from build123d import *

# Parameters (mm, degrees)
SKETCH1_R                      = 27.4955
SKETCH1_R_2                    = 2
SKETCH1_R_3                    = 52.3875
SKETCH1_R_4                    = 3.3
BOSS_EXTRUDE1_DEPTH            = 9.525
M8_CLEARANCE_HOLE1_D           = 9
M8_CLEARANCE_HOLE1_CSINK_D     = 9.05
M8_CLEARANCE_HOLE1_CSINK_ANGLE = 90
CIRPATTERN1_COUNT              = 9
CUT_EXTRUDE2_DEPTH             = 705.952403184


with BuildPart() as part:
    # Sketch1 → Boss-Extrude1 (new body)
    with BuildSketch(Plane(origin=(0, 0, 0), x_dir=(-1, 0, 0), z_dir=(0, 1, 0))):
        with BuildLine():
            Line((-663.918846707, 4.476573271), (-466.57213203, 18.457038772))
            ThreePointArc((-466.57213203, 18.457038772), (-464.265511177, 17.802436421), (-462.085988967, 16.80309317))
            ThreePointArc((-462.085988967, 16.80309317), (-454.417575787, 16.107140218), (-448.740207572, 21.308717033))
            Line((-448.740207572, 21.308717033), (-396.041564291, 141.567674451))
            ThreePointArc((-396.041564291, 141.567674451), (-393.869824608, 172.384252636), (-411.692336104, 197.617881552))
            ThreePointArc((-411.692336104, 197.617881552), (-413.372500119, 198.071242365), (-414.950136715, 197.336701751))
            Line((-414.950136715, 197.336701751), (-420.215020333, 192.071818133))
            ThreePointArc((-420.215020333, 192.071818133), (-427.298656721, 190.662795249), (-431.31121441, 196.668012211))
            Line((-431.31121441, 196.668012211), (-431.31121441, 203.240745001))
            ThreePointArc((-431.31121441, 203.240745001), (-431.968379704, 204.945600851), (-433.59982344, 205.768273949))
            ThreePointArc((-433.59982344, 205.768273949), (-438.15, 205.994), (-442.70017656, 205.768273949))
            ThreePointArc((-442.70017656, 205.768273949), (-444.331620296, 204.945600851), (-444.98878559, 203.240745001))
            Line((-444.98878559, 203.240745001), (-444.98878559, 196.668012211))
            ThreePointArc((-444.98878559, 196.668012211), (-451.48878559, 190.168012211), (-457.98878559, 196.668012211))
            Line((-457.98878559, 196.668012211), (-457.98878559, 197.245022653))
            ThreePointArc((-457.98878559, 197.245022653), (-459.278285753, 199.455870942), (-461.837486501, 199.421924563))
            ThreePointArc((-461.837486501, 199.421924563), (-464.019895008, 198.024699819), (-466.120112298, 196.506730383))
            Line((-466.120112298, 196.506730383), (-526.629683433, 150.121113421))
            ThreePointArc((-526.629683433, 150.121113421), (-551.530592574, 139.247052869), (-578.312485484, 134.661130809))
            ThreePointArc((-578.312485484, 134.661130809), (-599.244289514, 129.920579306), (-617.300018038, 118.318686532))
            ThreePointArc((-617.300018038, 118.318686532), (-626.772573796, 112.207783301), (-637.753125569, 109.658286556))
            Line((-637.753125569, 109.658286556), (-662.485690794, 106.73386739))
            ThreePointArc((-662.485690794, 106.73386739), (-670.168377129, 100.916938085), (-668.842832121, 91.372134981))
            Line((-668.842832121, 91.372134981), (-653.346537148, 71.746276485))
            ThreePointArc((-653.346537148, 71.746276485), (-651.347572908, 64.158994024), (-653.346537148, 56.571711562))
            Line((-653.346537148, 56.571711562), (-673.057822329, 18.34288652))
            ThreePointArc((-673.057822329, 18.34288652), (-672.544957076, 8.73610108), (-663.918846707, 4.476573271))
        make_face()
        with Locations(Location((-438.15, 160.02, 0), (0, 0, 270))):
            Circle(SKETCH1_R, mode=Mode.SUBTRACT)
        with Locations(Location((-632.402453753, 70.257452317, 0), (0, 0, 270))):
            Circle(SKETCH1_R_2, mode=Mode.SUBTRACT)
        with Locations(Location((-575.31, 72.821477372, 0), (0, 0, 270))):
            Circle(SKETCH1_R_3, mode=Mode.SUBTRACT)
        with Locations(Location((-661.367230642, 97.274762153, 0), (0, 0, 270))):
            Circle(SKETCH1_R_4, mode=Mode.SUBTRACT)
        with Locations(Location((-664.591931322, 13.977761728, 0), (0, 0, 270))):
            Circle(SKETCH1_R_4, mode=Mode.SUBTRACT)
        with Locations(Location((-457.464330992, 25.131712658, 0), (0, 0, 270))):
            Circle(SKETCH1_R_4, mode=Mode.SUBTRACT)
        with BuildLine():
            ThreePointArc((-518.217546247, 72.257452317), (-520.217546247, 70.257452317), (-518.217546247, 68.257452317))
            ThreePointArc((-518.217546247, 68.257452317), (-516.217546247, 70.257452317), (-518.217546247, 72.257452317))
        make_face(mode=Mode.SUBTRACT)
        with BuildLine():
            ThreePointArc((-575.31, 17.671477372), (-577.31, 15.671477372), (-575.31, 13.671477372))
            ThreePointArc((-575.31, 13.671477372), (-573.31, 15.671477372), (-575.31, 17.671477372))
        make_face(mode=Mode.SUBTRACT)
        with BuildLine():
            ThreePointArc((-575.31, 131.971477372), (-577.31, 129.971477372), (-575.31, 127.971477372))
            ThreePointArc((-575.31, 127.971477372), (-573.31, 129.971477372), (-575.31, 131.971477372))
        make_face(mode=Mode.SUBTRACT)
    extrude(amount=BOSS_EXTRUDE1_DEPTH)

    # M8 Clearance Hole1 (through all)
    with Locations(Plane(origin=(0, 0, 0), x_dir=(-1, 0, 0), z_dir=(0, -1, 0))):
        with Locations((-438.15, -199.019999978)):
            m8_clearance_hole1 = CounterSinkHole(M8_CLEARANCE_HOLE1_D / 2, M8_CLEARANCE_HOLE1_CSINK_D / 2, counter_sink_angle=M8_CLEARANCE_HOLE1_CSINK_ANGLE)

    # CirPattern1: M8 Clearance Hole1 ×9 about axis
    cirpattern1_axis = Axis((438.15, 0, 160.02), (0, 1, 0))
    for i in range(1, CIRPATTERN1_COUNT):
        add(m8_clearance_hole1.rotate(cirpattern1_axis, i * 360 / CIRPATTERN1_COUNT), mode=Mode.SUBTRACT)

    # Sketch10 → Cut-Extrude2 (cut, through all)
    with BuildSketch(Plane.XZ):
        with BuildLine():
            Line((459.226572507, 108.99771107), (501.653528527, 82.025066826))
            ThreePointArc((501.653528527, 82.025066826), (507.74174649, 75.794215969), (510.419523322, 67.504498748))
            ThreePointArc((510.419523322, 67.504498748), (511.358943513, 60.602369407), (513.030374645, 53.840105163))
            ThreePointArc((513.030374645, 53.840105163), (509.706018745, 36.414131356), (493.461745749, 29.283949023))
            Line((493.461745749, 29.283949023), (476.484388236, 30.486661525))
            ThreePointArc((476.484388236, 30.486661525), (470.70159957, 31.823239298), (465.610821582, 34.87464297))
            ThreePointArc((465.610821582, 34.87464297), (462.940510841, 36.590397323), (459.928151148, 37.590428091))
            ThreePointArc((459.928151148, 37.590428091), (455.812610468, 39.507256825), (453.051892844, 43.11146904))
            Line((453.051892844, 43.11146904), (434.678898983, 85.038868854))
            ThreePointArc((434.678898983, 85.038868854), (434.121445197, 98.905571071), (443.119806681, 109.470876354))
            ThreePointArc((443.119806681, 109.470876354), (446.028863873, 110.597089782), (449.124699442, 110.980198854))
            Line((449.124699442, 110.980198854), (452.412988142, 110.980198854))
            ThreePointArc((452.412988142, 110.980198854), (455.961057678, 110.474509108), (459.226572507, 108.99771107))
        make_face()
        with BuildLine():
            Line((488.447021855, 135.568616467), (518.5458141, 116.433517192))
            ThreePointArc((518.5458141, 116.433517192), (523.526027217, 115.31070897), (528.083819046, 117.610655627))
            ThreePointArc((528.083819046, 117.610655627), (531.194244853, 120.677331811), (534.503353276, 123.528481221))
            ThreePointArc((534.503353276, 123.528481221), (536.820485804, 129.284400418), (533.124064721, 134.267991506))
            ThreePointArc((533.124064721, 134.267991506), (526.661398117, 137.399578344), (520.391516426, 140.901217866))
            Line((520.391516426, 140.901217866), (497.676544793, 158.314132116))
            ThreePointArc((497.676544793, 158.314132116), (491.351665893, 159.127989595), (487.50938857, 154.038455032))
            ThreePointArc((487.50938857, 154.038455032), (486.663269024, 149.130057447), (485.330309415, 144.330942547))
            ThreePointArc((485.330309415, 144.330942547), (485.381225421, 139.4135911), (488.447021855, 135.568616467))
        make_face()
        with BuildLine():
            Line((639.635942668, 99.844305363), (644.459248163, 99.273989793))
            ThreePointArc((644.459248163, 99.273989793), (652.141934498, 93.457060489), (650.81638949, 83.912257385))
            Line((650.81638949, 83.912257385), (645.741529497, 77.485012402))
            ThreePointArc((645.741529497, 77.485012402), (642.355366484, 76.406104411), (640.089678042, 79.144132587))
            ThreePointArc((640.089678042, 79.144132587), (638.723930439, 87.486267946), (636.288558775, 95.581047358))
            ThreePointArc((636.288558775, 95.581047358), (636.765902184, 98.652013793), (639.635942668, 99.844305363))
        make_face()
        with BuildLine():
            Line((646.905882736, 48.27876498), (654.235681435, 34.063071304))
            ThreePointArc((654.235681435, 34.063071304), (653.551861098, 21.25402405), (642.050380606, 15.574653638))
            Line((642.050380606, 15.574653638), (626.09624364, 16.704878997))
            ThreePointArc((626.09624364, 16.704878997), (620.612206918, 20.775189015), (621.990747453, 27.464113323))
            ThreePointArc((621.990747453, 27.464113323), (629.655675988, 37.003462943), (635.399559362, 47.808930282))
            ThreePointArc((635.399559362, 47.808930282), (641.002883392, 51.713394678), (646.905882736, 48.27876498))
        make_face()
    extrude(amount=-CUT_EXTRUDE2_DEPTH, mode=Mode.SUBTRACT)


solid = part.part
Verification items for the finished model (mm, model axes). A direction names the side the tool comes from. Give positions to 0.01 mm unless a question says otherwise; leave off trailing zeros. Use one line per item in the form item = value. Start each with the question number.
Q1. Access from +Z, -Z, +X, -X, +Y, -Y to the whole of each face (thin tool, end or side, straight path). Record for faces 1 (the cylindrical face through (491.438, 4.696, 159.164)), 2 (the cylindrical face through (454.523, 4.696, 16.072)).
Q2. Go/stop test with flat-tipped pins: pin 1 Ø3.5 at (y, z) = (7, 199.5) entering from -X; pin 2 Ø0.6 at (y, z) = (5, 197) entering from -X; pin 3 Ø4 at (x, y) = (612.5, 4.5) entering from -Z. Record where each tip stops, or that it passes through.
Q3. Section check A-A (x = 438.15). Count the separate pieces of the cut face and the enclosed holes in it, then the cut area to 3 significant figures.
Q4. Scan lines: line 1 along X through (y, z) = (7, 105.5); line 2 along X through (y, z) = (7, 49.5); line 3 along X through (y, z) = (7, 72.5). Record each from-to range of solid material in increasing order. Write a range as [from, to].
Q5. Mould release check, pull along Z, two halves, no side actions. Record for faces 3 (the flat face through (496, 4.7, 173.6)), 4 (the cylindrical face through (395.247, 4.842, 166.594)), 5 (the flat face through (422.76, 4.7, 80.6)): +Z half, -Z half, draft (parallel to the pull), parting line (faces both ways), or undercut.
Evaluation:
q1.face_1 = +Y, -Y
q1.face_2 = -Z, +Y, -Y
q2.pin_1 = 411.9
q2.pin_2 = 410.43
q2.pin_3 = 7.98
q3.separate_pieces = 4
q3.enclosed_holes = 0
q3.area = 648 mm2
q4.line_1 = [411.85, 438.03], [464.73, 534.36], [616.26, 666.17]
q4.line_2 = [436.39, 450.25], [513.82, 528.4], [622.22, 636.44], [646.08, 656.99]
q4.line_3 = [426.31, 440.17], [509.32, 522.92], [627.7, 653.94]
q5.face_3 = +Z half
q5.face_4 = undercut
q5.face_5 = -Z half
